Source: CAD feature listing. Evaluate the final solid. Frame: model axes, mm. A direction names the side the tool comes from. Give positions to 0.01 mm unless a question says otherwise; leave off trailing zeros. Write each loop counter-clockwise with the first axis right and the second up, starting at its lowest first coordinate (ties: lowest second). Pieces come first, ordered by that corner, then holes. Notation, with made-up numbers: (23.5, 64) -> (28.5, 64) arc R23 cw to (28.5, 87) -> close; hole circle Ø2 at (22.25, 40.25). An arc over 180 degrees is marked (long way). Answer as a JSON object with one key per item and string values. Group by question number.
Item 1: Access query for faces 4 (the face through (-77, 57, 15)), 5 (the face through (-75, 0, -3)), 6 (the face through (-2, 33, 12)), 7 (the face through (-150, 27, -2)), 8 (the face through (-2, 84, 7)). Directions: +Z, -Z, +X, -X, +Y, -Y. A direction counts if a zero-diameter tool reaches every point of the face in a straight line with its end or side. Return the directions, or none.
Item 2: Section query A-A on y = 13. Return the cut outline in (x, z), plus the area to 4 significant figures.
Item 3: Section query D-D on x = -13.5. Return the cut outline in (y, z), plus the area to 3 significant figures.
Item 4: Section query B-B on z = -7.5. Return the cut outline in (x, y).
Item 5: Pull-direction query (Y, two-part tool) for faces 1 (the face through (-152.5, 55, -3)), 2 (the face through (-2, 79, 12)), 3 (the face through (-75, 112.5, -3)); classes: pulls with the +Y half, pulls with the -Y half, needs draft (parallel to the pull), parting line crosses it, or undercut.
Item 6: Ray query, probe 1 along Y at (x, z) = (-142.5, 16.4); probe 2 along X at (y, z) = (10, 18.85); probe 3 along Y at (x, z) = (-32, 4). Return the intervals inside material, ascending. Write a range as from..to.
Item 7: First-contact query: pin 1 Ø1.5 at (x, y) = (-142.5, 102.5) entering from +Z; pin 2 Ø3 at (x, y) = (-142.5, 10) entering from -Z. Flat tips, straight axial feed; report the tip coordinate or a pass-through.
Item 8: Section query C-C on y = 55. Return the cut outline in (x, z), plus the area to 4 significant figures.
Autodesk Fusion 360 part; units mm, degrees
sketch "Sketch1" plane through (0, 0, 0) normal (0, 0, 1) x (1, 0, 0)
  line L0 (0, 0) -> (-152.5, 0)
  line L1 (-152.5, 0) -> (-152.5, 112.5)
  line L2 (-152.5, 112.5) -> (0, 112.5)
  line L3 (0, 112.5) -> (0, 0)
  line L4 (-152.5, 112.5) -> (-147.5, 112.5)
  line L5 (0, 0) -> (0, 5)
  line L6 (-147.5, 107.5) -> (-5, 107.5)
  line L7 (-5, 107.5) -> (-5, 5)
  line L8 (-5, 5) -> (-147.5, 5)
  line L9 (-147.5, 5) -> (-147.5, 107.5)
  dimension "d1" = 152.5
  dimension "d2" = 112.5
  dimension "d3" = 5
  dimension "d4" = 5
  dimension "d5" = 5
  dimension "d6" = 5
extrude "Extrude1" add sketch "Sketch1" along normal blind 5 contours L0 L1 L2 L3 L4 L5 | L6 L7 L8 L9
sketch "Sketch2" plane through (0, 0, 0) normal (0, 0, -1) x (-1, 0, 0)
  line L0 (0, 0) -> (152.5, 0)
  line L1 (152.5, 0) -> (152.5, 112.5)
  line L2 (152.5, 112.5) -> (0, 112.5)
  line L3 (0, 112.5) -> (0, 0)
  line L4 (152.5, 112.5) -> (147.5, 112.5)
  line L5 (147.5, 112.5) -> (147.5, 107.5)
  line L6 (0, 0) -> (0, 5)
  line L7 (0, 5) -> (5, 5)
  line L8 (147.5, 107.5) -> (5, 107.5)
  line L9 (5, 107.5) -> (5, 5)
  line L10 (5, 5) -> (147.5, 5)
  line L11 (147.5, 5) -> (147.5, 107.5)
  dimension "d9" = 5
  dimension "d10" = 5
  dimension "d11" = 5
extrude "Extrude2" add sketch "Sketch2" along normal blind 25 contours L0 L1 L2 L3 L4 L5 L6 L7 L10 L11 | L2 L3 L5 L7 L8 L9
sketch "Sketch3" plane through (0, 0, 0) normal (1, 0, 0) x (0, 0, -1)
  line L0 (25, 112.5) -> (-5, 112.5)
  line L1 (-5, 112.5) -> (-5, 0)
  line L2 (-5, 0) -> (25, 0)
  line L3 (25, 0) -> (25, 112.5)
  line L4 (-5, 0) -> (-5, 20)
  line L5 (-5, 20) -> (-5, 45)
  line L6 (-5, 45) -> (-5, 70)
  line L7 (-5, 70) -> (10, 70)
  line L8 (-5, 45) -> (10, 45)
  line L9 (-5, 20) -> (10, 20)
  line L10 (10, 70) -> (10, 75)
  line L11 (10, 70) -> (10, 65)
  line L12 (10, 45) -> (10, 50)
  line L13 (10, 45) -> (10, 40)
  line L14 (10, 20) -> (10, 25)
  line L15 (10, 20) -> (10, 15)
  line L16 (10, 75) -> (5, 75)
  line L17 (10, 65) -> (15, 65)
  line L18 (10, 50) -> (5, 50)
  line L19 (10, 40) -> (15, 40)
  line L20 (10, 25) -> (5, 25)
  line L21 (10, 15) -> (15, 15)
  line L22 (5, 75) -> (15, 75)
  line L23 (15, 75) -> (15, 65)
  line L24 (15, 65) -> (5, 65)
  line L25 (5, 65) -> (5, 75)
  line L26 (5, 50) -> (15, 50)
  line L27 (15, 50) -> (15, 40)
  line L28 (15, 40) -> (5, 40)
  line L29 (5, 40) -> (5, 50)
  line L30 (5, 25) -> (15, 25)
  line L31 (15, 25) -> (15, 15)
  line L32 (15, 15) -> (5, 15)
  line L33 (5, 15) -> (5, 25)
  dimension "d14" = 25
  dimension "d15" = 5
  dimension "d16" = 5
  dimension "d17" = 5
  dimension "d18" = 5
  dimension "d19" = 5
  dimension "d20" = 5
  dimension "d21" = 5
  dimension "d22" = 5
  dimension "d23" = 5
  dimension "d24" = 5
extrude "Extrude3" cut sketch "Sketch3" against normal blind 10 contours L7 L10 L16 L22 L25 | L7 L11 L24 L25 | L8 L12 L18 L26 L29 | L8 L13 L28 L29 | L9 L14 L20 L30 L33 | L9 L15 L32 L33 | L10 L11 L17 L22 L23 L24 | L12 L13 L19 L26 L27 L28 | L14 L15 L21 L30 L31 L32
sketch "Sketch4" plane through (0, 0, 0) normal (0, 0, -1) x (-1, 0, 0)
  line L0 (147.5, 107.5) -> (5, 107.5)
  line L1 (5, 107.5) -> (5, 5)
  line L2 (5, 5) -> (147.5, 5)
  line L3 (147.5, 5) -> (147.5, 107.5)
  line L4 (5, 107.5) -> (5, 102.5)
  line L5 (5, 5) -> (5, 10)
  line L6 (10, 10) -> (142.5, 10)
  line L7 (10, 102.5) -> (142.5, 102.5)
  line L8 (142.5, 102.5) -> (142.5, 10)
  line L9 (10, 102.5) -> (10, 10)
  circle A0 centre (10, 102.5) radius 1.25
  circle A1 centre (10, 10) radius 1.25
  circle A2 centre (142.5, 10) radius 1.25
  circle A3 centre (142.5, 102.5) radius 1.25
  dimension "d27" = 5
  dimension "d28" = 132.5
  dimension "d29" = 132.5
  dimension "d30" = 2.5
  dimension "d31" = 2.5
  dimension "d32" = 2.5
  dimension "d33" = 2.5
extrude "Extrude4" cut sketch "Sketch4" against normal blind 20 contours L6 L9 A1 | L6 L9 A1 | L6 L8 A2 | L6 L8 A2 | L7 L9 A0 | L7 L9 A0 | L7 L8 A3 | L7 L8 A3
extrude "Extrude5" add 1 faces at (-54.5498, 41.1167, 5) along direction (0, 0, 1) blind 10
sketch "Sketch5" plane through (0, 0, 0) normal (1, 0, 0) x (0, 0, -1)
  line L0 (15, 25) -> (15, 15)
  line L1 (15, 15) -> (5, 15)
  line L2 (5, 15) -> (5, 25)
  line L3 (5, 25) -> (15, 25)
  line L4 (15, 50) -> (15, 40)
  line L5 (15, 40) -> (5, 40)
  line L6 (5, 40) -> (5, 50)
  line L7 (5, 50) -> (15, 50)
  line L8 (15, 75) -> (15, 65)
  line L9 (15, 65) -> (5, 65)
  line L10 (5, 65) -> (5, 75)
  line L11 (5, 75) -> (15, 75)
  line L12 (25, 112.5) -> (-15, 112.5)
  line L13 (-15, 112.5) -> (-15, 0)
  line L14 (-15, 0) -> (25, 0)
  line L15 (25, 0) -> (25, 112.5)
  line L16 (25, 112.5) -> (22.5, 112.5)
  line L17 (22.5, 112.5) -> (22.5, 110)
  line L18 (25, 0) -> (22.5, 0)
  line L19 (22.5, 0) -> (22.5, 2.5)
  line L20 (22.5, 110) -> (20, 110)
  line L21 (22.5, 2.5) -> (20, 2.5)
  line L22 (22.5, 110) -> (20, 110)
  line L23 (20, 110) -> (20, 2.5)
  line L24 (20, 2.5) -> (22.5, 2.5)
  line L25 (22.5, 2.5) -> (22.5, 110)
  dimension "d38" = 2.5
  dimension "d39" = 2.5
  dimension "d40" = 2.5
extrude "Extrude6" cut sketch "Sketch5" against normal blind 150.5 contours L20 L21 L22 L23 L24 L25
extrude "Extrude7" cut 1 faces at (-147.5, 39.1667, -23.3333) along direction (-1, 0, 0) blind 1
extrude "Extrude8" cut 1 faces at (-148.5, 39.1667, -23.3333) along direction (-1, 0, 0) blind 1
extrude "Extrude9" cut 1 faces at (-150.5, 74.1667, -20.8333) along direction (-1, 0, 0) blind 1
extrude "Extrude10" cut 1 faces at (-101.3333, 107.5, -23.3333) along direction (0, 1, 0) blind 3
extrude "Extrude11" cut 1 faces at (-53.1667, 5, -24.1667) along direction (0, -1, 0) blind 3
extrude "Extrude12" add 1 faces at (-54.5498, 41.1167, 15) along direction (0, 0, 1) blind 5
extrude "Extrude13" cut 1 faces at (-54.5555, 41.0963, 0) along direction (0, 0, 1) blind 15
sketch "Sketch6" plane through (0, 0, 0) normal (1, 0, 0) x (0, 0, -1)
  line L0 (20, 110) -> (22.5, 110)
  line L1 (22.5, 110) -> (22.5, 2.5)
  line L2 (22.5, 2.5) -> (20, 2.5)
  line L3 (20, 2.5) -> (20, 110)
  line L4 (15, 25) -> (15, 15)
  line L5 (15, 15) -> (5, 15)
  line L6 (5, 15) -> (5, 25)
  line L7 (5, 25) -> (15, 25)
  line L8 (15, 50) -> (15, 40)
  line L9 (15, 40) -> (5, 40)
  line L10 (5, 40) -> (5, 50)
  line L11 (5, 50) -> (15, 50)
  line L12 (15, 75) -> (15, 65)
  line L13 (15, 65) -> (5, 65)
  line L14 (5, 65) -> (5, 75)
  line L15 (5, 75) -> (15, 75)
  line L16 (25, 112.5) -> (-20, 112.5)
  line L17 (-20, 112.5) -> (-20, 0)
  line L18 (-20, 0) -> (25, 0)
  line L19 (25, 0) -> (25, 112.5)
sketch "Sketch7" plane through (0, 0, 0) normal (1, 0, 0) x (0, 0, -1)
sketch "Sketch8" plane through (0, 0, 0) normal (1, 0, 0) x (0, 0, -1)
  line L0 (-14, 84) -> (-4, 84)
  line L1 (-4, 84) -> (-4, 74)
  line L2 (-4, 74) -> (-14, 74)
  line L3 (-14, 74) -> (-14, 84)
  line L4 (-14, 62) -> (-4, 62)
  line L5 (-4, 62) -> (-4, 52)
  line L6 (-4, 52) -> (-14, 52)
  line L7 (-14, 52) -> (-14, 62)
  line L8 (-14, 38) -> (-4, 38)
  line L9 (-4, 38) -> (-4, 28)
  line L10 (-4, 28) -> (-14, 28)
  line L11 (-14, 28) -> (-14, 38)
extrude "Extrude14" add sketch "Sketch6" against normal blind 5 contours L4 L5 L6 L7 | L8 L9 L10 L11 | L12 L13 L14 L15
extrude "Extrude15" cut sketch "Sketch8" against normal blind 5
sketch "Sketch9" plane through (-152.5, 0, 0) normal (-1, 0, 0) x (0, 0, 1)
  line L0 (-25, 0) -> (20, 0)
  line L1 (20, 0) -> (20, 112.5)
  line L2 (20, 112.5) -> (-25, 112.5)
  line L3 (-25, 112.5) -> (-25, 0)
  line L4 (12, 15) -> (-2, 15)
  line L5 (-2, 15) -> (-2, 40)
  line L6 (-2, 40) -> (12, 40)
  line L7 (12, 40) -> (12, 15)
extrude "Extrude16" cut sketch "Sketch9" against normal blind 5 contours L4 L5 L6 L7
sketch "Sketch10" plane through (0, 0, 0) normal (1, 0, 0) x (0, 0, -1)
  line L0 (-4, 84) -> (-4, 74)
  line L1 (-4, 74) -> (-14, 74)
  line L2 (-14, 74) -> (-14, 84)
  line L3 (-14, 84) -> (-4, 84)
  line L4 (-4, 62) -> (-4, 52)
  line L5 (-4, 52) -> (-14, 52)
  line L6 (-14, 52) -> (-14, 62)
  line L7 (-14, 62) -> (-4, 62)
  line L8 (-4, 38) -> (-4, 28)
  line L9 (-4, 28) -> (-14, 28)
  line L10 (-14, 28) -> (-14, 38)
  line L11 (-14, 38) -> (-4, 38)
  line L12 (20, 110) -> (22.5, 110)
  line L13 (22.5, 110) -> (22.5, 2.5)
  line L14 (22.5, 2.5) -> (20, 2.5)
  line L15 (20, 2.5) -> (20, 110)
  line L16 (25, 112.5) -> (-20, 112.5)
  line L17 (-20, 112.5) -> (-20, 0)
  line L18 (-20, 0) -> (25, 0)
  line L19 (25, 0) -> (25, 112.5)
  line L20 (-4, 84) -> (-2, 84)
  line L21 (-2, 84) -> (-2, 74)
  line L22 (-2, 74) -> (-4, 74)
  line L23 (-4, 74) -> (-4, 84)
  line L24 (-4, 62) -> (-2, 62)
  line L25 (-2, 62) -> (-2, 52)
  line L26 (-2, 52) -> (-4, 52)
  line L27 (-4, 52) -> (-4, 62)
  line L28 (-4, 38) -> (-2, 38)
  line L29 (-2, 38) -> (-2, 28)
  line L30 (-2, 28) -> (-4, 28)
  line L31 (-4, 28) -> (-4, 38)
  line L32 (-14, 28) -> (-12, 28)
  line L33 (-12, 28) -> (-12, 84)
  line L34 (-12, 84) -> (-14, 84)
  line L35 (-14, 84) -> (-14, 28)
extrude "Extrude17" add sketch "Sketch10" against normal blind 5 contours L1 L2 L3 L33 L34 L35 | L5 L6 L7 L33 L35 | L9 L10 L11 L32 L33 L35
sketch "Sketch11" plane through (0, 0, 0) normal (1, 0, 0) x (0, 0, -1)
  line L0 (-4, 84) -> (-4, 74)
  line L1 (-4, 74) -> (-12, 74)
  line L2 (-12, 74) -> (-12, 84)
  line L3 (-12, 84) -> (-4, 84)
  line L4 (-4, 62) -> (-4, 52)
  line L5 (-4, 52) -> (-12, 52)
  line L6 (-12, 52) -> (-12, 62)
  line L7 (-12, 62) -> (-4, 62)
  line L8 (-4, 38) -> (-4, 28)
  line L9 (-4, 28) -> (-12, 28)
  line L10 (-12, 28) -> (-12, 38)
  line L11 (-12, 38) -> (-4, 38)
  line L12 (20, 110) -> (22.5, 110)
  line L13 (22.5, 110) -> (22.5, 2.5)
  line L14 (22.5, 2.5) -> (20, 2.5)
  line L15 (20, 2.5) -> (20, 110)
  line L16 (25, 112.5) -> (-20, 112.5)
  line L17 (-20, 112.5) -> (-20, 0)
  line L18 (-20, 0) -> (25, 0)
  line L19 (25, 0) -> (25, 112.5)
  line L20 (-4, 62) -> (-2, 62)
  line L21 (-2, 62) -> (-2, 52)
  line L22 (-2, 52) -> (-4, 52)
  line L23 (-4, 52) -> (-4, 62)
  line L24 (-4, 38) -> (-2, 38)
  line L25 (-2, 38) -> (-2, 28)
  line L26 (-2, 28) -> (-4, 28)
  line L27 (-4, 28) -> (-4, 38)
  line L28 (-4, 84) -> (-2, 84)
  line L29 (-2, 84) -> (-2, 74)
  line L30 (-2, 74) -> (-4, 74)
  line L31 (-4, 74) -> (-4, 84)
extrude "Extrude18" cut sketch "Sketch11" against normal blind 5 contours L0 L28 L29 L30 L31 | L4 L20 L21 L22 L23 | L8 L24 L25 L26 L27
Worked answers:
{
 "1": {"face 4": "-Z", "face 5": "+Z, -Z, +X, -X, -Y", "face 6": "+X, -X", "face 7": "-X", "face 8": "+X"},
 "2": {"outline": "(-152.5, -25) -> (-149.5, -25) -> (-149.5, -22.5) -> (-151.5, -22.5) -> (-151.5, -20) -> (-147.5, -20) -> (-147.5, 15) -> (-5, 15) -> (-5, -20) -> (0, -20) -> (0, 20) -> (-152.5, 20) -> close; (-5, -25) -> (0, -25) -> (0, -22.5) -> (-5, -22.5) -> close", "area": "1,135 mm^2"},
 "3": {"outline": "(0, -25) -> (2, -25) -> (2, -22.5) -> (2.5, -22.5) -> (2.5, -20) -> (5, -20) -> (5, 15) -> (107.5, 15) -> (107.5, -20) -> (110, -20) -> (110, -22.5) -> (110.5, -22.5) -> (110.5, -25) -> (112.5, -25) -> (112.5, 20) -> (0, 20) -> close", "area": "935 mm^2"},
 "4": {"outline": "(-152.5, 0) -> (0, 0) -> (0, 112.5) -> (-152.5, 112.5) -> close; hole (-147.5, 5) -> (-5, 5) -> (-5, 107.5) -> (-147.5, 107.5) -> close"},
 "5": {"face 1": "needs draft", "face 2": "undercut", "face 3": "pulls with the +Y half"},
 "6": {"probe 1": "0..8.75, 11.25..101.25, 103.75..112.5", "probe 2": "-152.5..-143.75, -141.25..-11.25, -8.75..0", "probe 3": "0..5, 107.5..112.5"},
 "7": {"pin 1": "through", "pin 2": "z = 15"},
 "8": {"outline": "(-152.5, -25) -> (-149.5, -25) -> (-149.5, -22.5) -> (-151.5, -22.5) -> (-151.5, -20) -> (-147.5, -20) -> (-147.5, 15) -> (-5, 15) -> (-5, 12) -> (0, 12) -> (0, 20) -> (-152.5, 20) -> close; (-5, -25) -> (0, -25) -> (0, -22.5) -> (-5, -22.5) -> close; (-5, -20) -> (0, -20) -> (0, 2) -> (-5, 2) -> close", "area": "1,085 mm^2"}
}
